Design review of the part built by this model. Coordinates are the model's own, in mm. A direction names the side the tool comes from. Round coordinates to 2 decimals unless told otherwise and drop trailing zeros. Write each loop counter-clockwise with the first axis right and the second up, starting at its lowest first coordinate (ties: lowest second). Pieces come first, ordered by that corner, then holes.
from build123d import *

# Parameters (mm, degrees)
SKETCH_1_W          = 200
SKETCH_1_H          = 250
SKETCH_1_R          = 4
EXTRUDE_1_DEPTH     = 10
EXTRUDE_START       = -15
SKETCH_2_R          = 4
EXTRUDE_3_DEPTH     = 15
CUT_EXTRUDE_1_DEPTH = 0.2
SKETCH_4_R          = 1.525
CUT_EXTRUDE_2_DEPTH = 321.507410211
SKETCH_5_R          = 1.5
CUT_EXTRUDE_3_DEPTH = 321.507410211
SKETCH_6_R          = 1.75
CUT_EXTRUDE_4_DEPTH = 321.507410211
SKETCH_7_R          = 1.5
CUT_EXTRUDE_5_DEPTH = 321.507410211


with BuildPart() as part:
    # 草图1 → 凸台-拉伸1 (new body)
    with BuildSketch(Plane(origin=(0, 0, 0), x_dir=(1, 0, 0), z_dir=(0, 1, 0))):
        with Locations((100, -125)):
            Rectangle(SKETCH_1_W, SKETCH_1_H)
        with Locations(Location((180, -15, 0), (0, 0, 270))):
            Circle(SKETCH_1_R, mode=Mode.SUBTRACT)
        with Locations(Location((180, -235, 0), (0, 0, 90))):
            Circle(SKETCH_1_R, mode=Mode.SUBTRACT)
        with Locations(Location((20, -15, 0), (0, 0, 90))):
            Circle(SKETCH_1_R, mode=Mode.SUBTRACT)
        with Locations(Location((20, -235, 0), (0, 0, 270))):
            Circle(SKETCH_1_R, mode=Mode.SUBTRACT)
    extrude(amount=EXTRUDE_1_DEPTH)

    # 草图2 → 凸台-拉伸3 (add)
    with BuildSketch(Plane(origin=(0, 10, 0), x_dir=(1, 0, 0), z_dir=(0, 1, 0)).offset(EXTRUDE_START)):
        with Locations(Location((180, -235, 0), (0, 0, 270))):
            Circle(SKETCH_2_R)
        with Locations(Location((20, -235, 0), (0, 0, 270))):
            Circle(SKETCH_2_R)
        with Locations(Location((180, -15, 0), (0, 0, 270))):
            Circle(SKETCH_2_R)
        with Locations(Location((20, -15, 0), (0, 0, 270))):
            Circle(SKETCH_2_R)
    extrude(amount=EXTRUDE_3_DEPTH)

    # 草图3 → 切除-拉伸1 (cut)
    with BuildSketch(Plane(origin=(0, 10, 0), x_dir=(1, 0, 0), z_dir=(0, 1, 0))):
        Polygon((56, -240), (53, -234.803847577), (47, -234.803847577), (44, -240), (47, -245.196152423), (53, -245.196152423), align=None)
        Polygon((147, -245.196152423), (144, -240), (147, -234.803847577), (153, -234.803847577), (156, -240), (153, -245.196152423), align=None)
        Polygon((144, -10), (147, -15.196152423), (153, -15.196152423), (156, -10), (153, -4.803847577), (147, -4.803847577), align=None)
        Polygon((53, -4.803847577), (56, -10), (53, -15.196152423), (47, -15.196152423), (44, -10), (47, -4.803847577), align=None)
    extrude(amount=-CUT_EXTRUDE_1_DEPTH, mode=Mode.SUBTRACT)

    # 草图4 → 切除-拉伸2 (cut, through all)
    with BuildSketch(Plane(origin=(0, 10, 0), x_dir=(1, 0, 0), z_dir=(0, 1, 0))):
        with Locations(Location((150, -10, 0), (0, 0, 270))):
            Circle(SKETCH_4_R)
        with Locations(Location((50, -10, 0), (0, 0, 270))):
            Circle(SKETCH_4_R)
        with Locations(Location((50, -240, 0), (0, 0, 270))):
            Circle(SKETCH_4_R)
        with Locations(Location((150, -240, 0), (0, 0, 270))):
            Circle(SKETCH_4_R)
    extrude(amount=-CUT_EXTRUDE_2_DEPTH, mode=Mode.SUBTRACT)

    # 草图5 → 切除-拉伸3 (cut, through all)
    with BuildSketch(Plane(origin=(0, 10, 0), x_dir=(1, 0, 0), z_dir=(0, 1, 0))):
        with Locations(Location((69.6, -68.863237915, 0), (0, 0, 270))):
            Circle(SKETCH_5_R)
        with Locations(Location((69.6, -108.363237915, 0), (0, 0, 270))):
            Circle(SKETCH_5_R)
        with Locations(Location((130.4, -108.363237915, 0), (0, 0, 270))):
            Circle(SKETCH_5_R)
        with Locations(Location((130.4, -68.863237915, 0), (0, 0, 270))):
            Circle(SKETCH_5_R)
    extrude(amount=-CUT_EXTRUDE_3_DEPTH, mode=Mode.SUBTRACT)

    # 草图6 → 切除-拉伸4 (cut, through all)
    with BuildSketch(Plane(origin=(0, 10, 0), x_dir=(1, 0, 0), z_dir=(0, 1, 0))):
        with Locations(Location((190, -54, 0), (0, 0, 270))):
            Circle(SKETCH_6_R)
        with Locations(Location((160, -54, 0), (0, 0, 270))):
            Circle(SKETCH_6_R)
        with Locations(Location((160, -30, 0), (0, 0, 270))):
            Circle(SKETCH_6_R)
        with Locations(Location((190, -30, 0), (0, 0, 270))):
            Circle(SKETCH_6_R)
        with Locations(Location((190, -220, 0), (0, 0, 270))):
            Circle(SKETCH_6_R)
        with Locations(Location((160, -220, 0), (0, 0, 270))):
            Circle(SKETCH_6_R)
        with Locations(Location((160, -196, 0), (0, 0, 270))):
            Circle(SKETCH_6_R)
        with Locations(Location((190, -196, 0), (0, 0, 270))):
            Circle(SKETCH_6_R)
        with Locations(Location((40, -54, 0), (0, 0, 270))):
            Circle(SKETCH_6_R)
        with Locations(Location((10, -54, 0), (0, 0, 270))):
            Circle(SKETCH_6_R)
        with Locations(Location((10, -30, 0), (0, 0, 270))):
            Circle(SKETCH_6_R)
        with Locations(Location((40, -30, 0), (0, 0, 270))):
            Circle(SKETCH_6_R)
        with Locations(Location((40, -220, 0), (0, 0, 270))):
            Circle(SKETCH_6_R)
        with Locations(Location((10, -220, 0), (0, 0, 270))):
            Circle(SKETCH_6_R)
        with Locations(Location((10, -196, 0), (0, 0, 270))):
            Circle(SKETCH_6_R)
        with Locations(Location((40, -196, 0), (0, 0, 270))):
            Circle(SKETCH_6_R)
    extrude(amount=-CUT_EXTRUDE_4_DEPTH, mode=Mode.SUBTRACT)

    # 草图7 → 切除-拉伸5 (cut, through all)
    with BuildSketch(Plane(origin=(0, 10, 0), x_dir=(1, 0, 0), z_dir=(0, 1, 0))):
        with Locations(Location((121.65, -205, 0), (0, 0, 270))):
            Circle(SKETCH_7_R)
        with Locations(Location((78.35, -205, 0), (0, 0, 270))):
            Circle(SKETCH_7_R)
    extrude(amount=-CUT_EXTRUDE_5_DEPTH, mode=Mode.SUBTRACT)


solid = part.part
1) For P1, Ø4, axis at x = 121.65, z = 205, coming from the +Y side; P2, Ø3, axis at x = 43.5, z = 172.5, coming from the -Y side; P3, Ø4, axis at x = 50, z = 10, coming from the +Y side; P4, Ø2, axis at x = 160, z = 196, coming from the +Y side, all flat-tipped, find the tip position at first contact; note any pin that passes through.
2) Add section A-A on x = 20. State the section outline as (y, z) points.
3) The part is to be moulded in two halves that separate along Z. For faces 4 (the face through (99, 5, 250)), 5 (the face through (20, -5, 15)), 6 (the face through (183.966, -2.535, 14.479)), say which applies: pulls with the +Z half, pulls with the -Z half, needs draft (parallel to the pull), parting line crosses it, or undercut.
4) Add section C-C on x = 111.5. State the section outline as (y, z) points.
5) For line 1 along Z through (x, y) = (160, 7.75); line 2 along Z through (x, y) = (130.4, 2); line 3 along X through (y, z) = (7.75, 220), list the stretches that pass through material, from the lowest coordinate up.
6) Add section B-B on z = 182.5. State the section outline as (x, y) points, and give its area (3 significant figures).
7) For faces 1 (the face through (182.7, -2.54, 232.05)), 2 (the face through (148.8, 9.8, 238.8)), 3 (the face through (0, 5, 127)), list the 3-axis set-ups (+Z, -Z, +X, -X, +Y, -Y) from which the entire face can be reached by the end or side of a thin tool; tool diameter is ignored.
Computed:
1. P1: stops at y = 10
1. P2: stops at y = 0
1. P3: stops at y = 9.8
1. P4: passes through
2. outline: (-5, 11) - (0, 11) - (0, 0) - (10, 0) - (10, 250) - (0, 250) - (0, 239) - (-5, 239) - (-5, 231) - (0, 231) - (0, 19) - (-5, 19) - close
3. face 4: pulls with the +Z half
3. face 5: needs draft
3. face 6: undercut
4. outline: (0, 0) - (10, 0) - (10, 250) - (0, 250) - close
5. line 1: z = 0 to 28.25, 31.75 to 52.25, 55.75 to 194.25, 197.75 to 218.25, 221.75 to 250
5. line 2: z = 0 to 67.36, 70.36 to 106.86, 109.86 to 250
5. line 3: x = 0 to 8.25, 11.75 to 38.25, 41.75 to 158.25, 161.75 to 188.25, 191.75 to 200
6. outline: (0, 0) - (200, 0) - (200, 10) - (0, 10) - close
6. area: 2,000 mm2
7. face 1: -Y
7. face 2: +Y
7. face 3: +Z, -Z, -X, +Y, -Y
